The model under review builds one solid part; all positions refer to its coordinate system, in mm. A direction names the side the tool comes from. Round coordinates to 2 decimals unless told otherwise and drop trailing zeros. Loops run counter-clockwise (first coordinate to the right, second up) from the corner with the lowest first, then second, coordinate; pieces in that order, holes last. Notation, with made-up numbers: M -8,-11 L 18,-11 A23 ccw 18,3 Z; hole C 31.25,-28 d3. An arc over 180 degrees is marked long. Answer as a JSON object with one key per item and string values. Group by question number.
Item 1: Insertion check: P1, Ø1.5, axis at x = 5, y = -7, coming from the +Z side; P2, Ø2, axis at x = 5, z = -6.5, coming from the +Y side; P3, Ø5, axis at y = 0, z = 13, coming from the +X side. Each pin has a flat end and moves straight along its axis. Give the tip position at first contact, or say it passes through.
Item 2: Consider section C-C (x = 1.25). Give the boundary of the cut face in (y, z), and give its area (3 significant figures).
Item 3: Consider section A-A (y = 0). Give the boundary of the cut face in (x, z).
Item 4: The part is to be moulded in two halves that separate along Y. For faces 1 (the face through (6.042, 7.964, 2.508)), 2 (the face through (0, 0, -8)), 3 (the face through (1.5, -14.6, -1.2)), say which applies: +Y half, -Y half, draft (parallel to the pull), parting line (faces both ways), or undercut.
Item 5: Consider section D-D (z = -12.5). Give the boundary of the cut face in (x, y).
Item 6: To check wall thickness, follow line 1 (Z direction, x = 2.2, y = 0); line 2 (Z direction, x = 4.5, y = 0); line 3 (X direction, y = -2.5, z = 4). State the ranges of each line that lie inside material, in increasing order.
Item 7: Tool access review of faces 4 (the face through (7.5, 0, 0)), 5 (the face through (3, 8, -4)), 6 (the face through (1, 0, 15)): name each direction out of +Z, -Z, +X, -X, +Y, -Y from which nothing blocks a thin tool from reaching the whole face with its end or side.
```python
from build123d import *

# Parameters (mm, degrees)
F0_R     = 17.5
F0_R_2   = 2
F0_R_3   = 6.35
F1_DEPTH = 9
F2_R     = 17.5
F2_R_2   = 8.35
F3_DEPTH = 6
F4_R     = 6.4
F5_DEPTH = 1.5


with BuildPart() as f1:
    # F0 (on Right) → F1 (new body)
    with BuildSketch(Plane.YZ):
        Circle(F0_R)
        with Locations((0, -13)):
            Circle(F0_R_2, mode=Mode.SUBTRACT)
        with Locations((-13, 0)):
            Circle(F0_R_2, mode=Mode.SUBTRACT)
        Circle(F0_R_3, mode=Mode.SUBTRACT)
        with Locations((13, 0)):
            Circle(F0_R_2, mode=Mode.SUBTRACT)
        with Locations((0, 13)):
            Circle(F0_R_2, mode=Mode.SUBTRACT)
    extrude(amount=F1_DEPTH)

    # F2 (on face) → F3 (cut)
    with BuildSketch(Plane.YZ.offset(9)):
        Circle(F2_R)
        Circle(F2_R_2, mode=Mode.SUBTRACT)
    extrude(amount=-F3_DEPTH, mode=Mode.SUBTRACT)

    # F4 (on face) → F5 (join)
    with BuildSketch(Plane.YZ.offset(9)):
        Circle(F4_R)
    extrude(amount=-F5_DEPTH)


solid = f1.part
```
Geometry results:
{
 "1": {"P1": "stops at z = 5.54", "P2": "stops at y = 6.28", "P3": "stops at x = 3"},
 "2": {"outline": "C 0,0 d35; hole C -13,0 d4; hole C 0,0 d12.7; hole C 0,-13 d4; hole C 0,13 d4; hole C 13,0 d4", "area": "785 mm^2"},
 "3": {"outline": "M 0,-17.5 L 3,-17.5 L 3,-15 L 0,-15 Z; M 0,-11 L 3,-11 L 3,-8.35 L 9,-8.35 L 9,8.35 L 3,8.35 L 3,11 L 0,11 L 0,6.35 L 7.5,6.35 L 7.5,-6.35 L 0,-6.35 Z; M 0,15 L 3,15 L 3,17.5 L 0,17.5 Z"},
 "4": {"face 1": "parting line", "face 2": "draft", "face 3": "undercut"},
 "5": {"outline": "M 0,-12.25 L 3,-12.25 L 3,-1.94 L 0,-1.94 Z; M 0,1.94 L 3,1.94 L 3,12.25 L 0,12.25 Z"},
 "6": {"line 1": "z = -17.5 to -15, -11 to -6.35, 6.35 to 11, 15 to 17.5", "line 2": "z = -8.35 to -6.35, 6.35 to 8.35", "line 3": "x = 7.5 to 9"},
 "7": {"face 4": "-X", "face 5": "+X", "face 6": "+X, -X"}
}
